Work out the finished part from the listing and answer in its coordinate system (mm). A direction names the side the tool comes from. Give positions to 0.01 mm unless a question says otherwise; leave off trailing zeros. Order: outer loops, then holes, each group sorted by start corner. A loop starts at its lowest first (then second) coordinate and runs counter-clockwise, first axis right, second up. Notation, with made-up numbers: M 84.5,56 L 120.5,56 A19 ccw 120.5,65 Z; hole C 56.25,-20 d2. An arc over 180 degrees is marked long. One line per item, written item: value.
from build123d import *

# Parameters (mm, degrees)
CROQUIS1_R              = 45
SALIENTE_EXTRUIR1_DEPTH = 8
CROQUIS2_R              = 8
SALIENTE_EXTRUIR2_DEPTH = 10
REDONDEO1_R             = 3


with BuildPart() as part:
    # Croquis1 → Saliente-Extruir1 (new body)
    with BuildSketch(Plane.XY):
        Circle(CROQUIS1_R)
    extrude(amount=SALIENTE_EXTRUIR1_DEPTH)

    # Croquis2 → Saliente-Extruir2 (add)
    with BuildSketch(Plane.XY.offset(8)):
        Circle(CROQUIS2_R)
    extrude(amount=SALIENTE_EXTRUIR2_DEPTH)

    # Redondeo1
    redondeo1_edges = [part.edges().sort_by_distance(p)[0] for p in [
        (-45, 0, 0),
        (-45, 0, 8),
    ]]
    fillet(redondeo1_edges, radius=REDONDEO1_R)


solid = part.part
(1) Given P1, Ø8, axis at x = -20.5, y = 8, coming from the +Z side; P2, Ø10, axis at y = -2, z = 12, coming from the +X side; P3, Ø1, axis at y = 32, z = 9, coming from the +X side; P4, Ø5, axis at y = 29, z = 8, coming from the +X side, each flat-ended and moving along its own axis, determine where each tip first touches the part or whether it passes through.
Findings:
P1: stops at z = 8
P2: stops at x = 44.2
P3: passes through
P4: stops at x = 35.51
(2) Find the intervals of material crossed by probe 1 along Z at (x, y) = (-23.5, -0.5); probe 2 along Y at (x, z) = (-29, 1); probe 3 along Y at (x, z) = (-8, 7.25), in increasing order. Write a range as from..to.
Findings:
probe 1: z = 0..8
probe 2: y = -33.4..33.4
probe 3: y = -43.25..43.25
(3) Section D-D, the plane z = 6.5 is taken. Give the vertices of the cut face in (x, y), then the cut area to 3 significant figures.
Findings:
outline: C 0,0 d89.2
area: 6,250 mm^2
(4) Which of the six approach directions +Z, -Z, +X, -X, +Y, -Y give full straight-line access (tool end or side, diameter ignored) to faces 1 (the flat face through (-1, 1, 0)), 2 (the cylindrical face through (-1.73, -7.81, 12.93))?
Findings:
face 1: -Z, +X, -X, +Y, -Y
face 2: +Z
(5) Section C-C, the plane z = 11.5 is taken. Give the vertices of the cut face in (x, y), then the cut area to 3 significant figures.
Findings:
outline: C 0,0 d16
area: 201 mm^2
(6) Section A-A, the plane y = 0 is taken. Give the vertices of the cut face in (x, z), then the cut area to 3 significant figures.
Findings:
outline: M -45,3 A3 ccw -42,0 L 42,0 A3 ccw 45,3 L 45,5 A3 ccw 42,8 L 8,8 L 8,18 L -8,18 L -8,8 L -42,8 A3 ccw -45,5 Z
area: 872 mm^2
